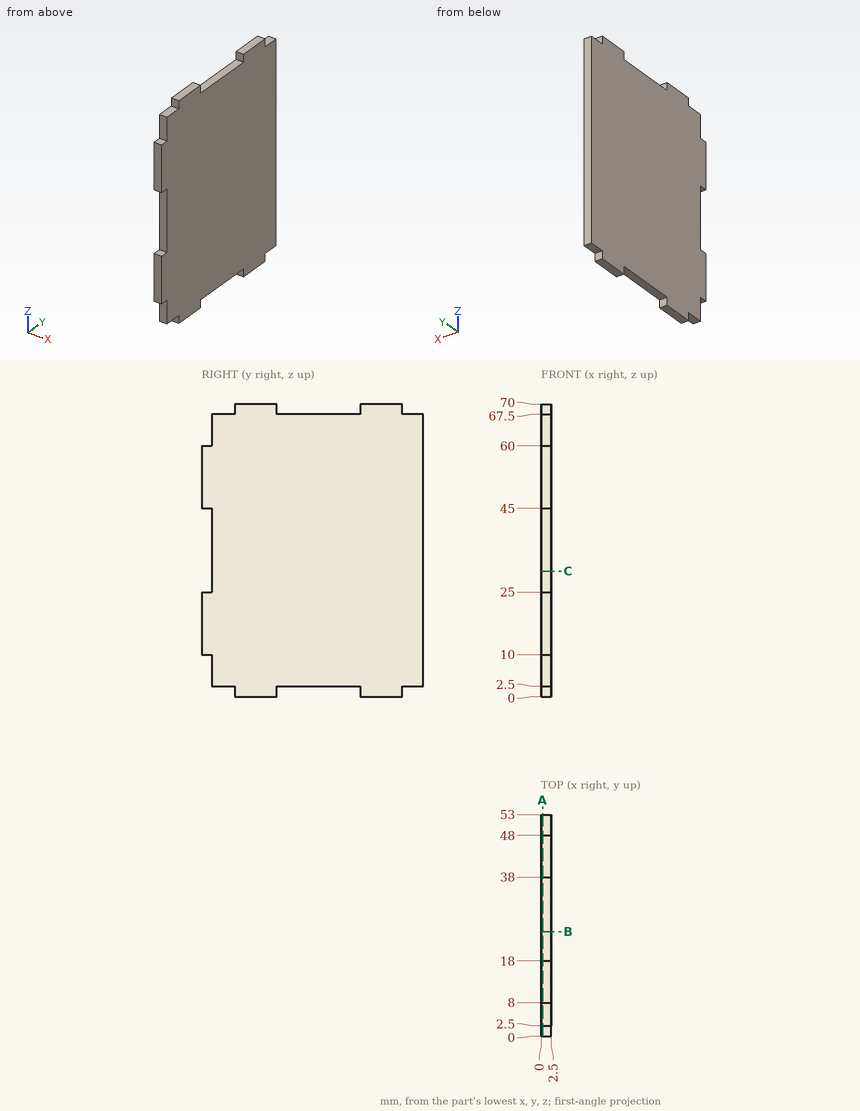
Design review of the part shown in the three views and the two pictorial views. Dimensions are in mm from the part's minimum x, y and z. Give positions to 0.01 mm unless a question says otherwise; leave off trailing zeros. Loops run counter-clockwise (first coordinate to the right, second up) from the corner with the lowest first, then second, coordinate; pieces in that order, holes last. Notation, with made-up numbers: M -15.5,85 L 3.5,85 A15 cw 3.5,99 Z; hole C 54.5,-30.75 d8. An arc over 180 degrees is marked long. Put each result on its own line as item: value. Start each with the question number.
(1) For pin 1 (1.2 mm diameter, centred on x = 1.5, z = 68.5, fed in from -Y); pin 2 (0.8 mm diameter, centred on x = 1.5, z = 0.5, fed in from +Y); pin 3 (1.2 mm diameter, centred on x = 1.5, y = 1, fed in from +Z), all flat-tipped, find the tip position at first contact; note any pin that passes through.
(2) Wall thickness on L1, parallel to Z at x = 1.15, y = 29; L2, parallel to Y at x = 1.55, z = 31: over which ranges is each line inside the solid? List them lowest first.
(3) Add section C-C, the plane z = 30. Write out the cut boundary in (x, y), then the cut area to 3 significant figures.
(4) Add section B-B, the plane y = 25. Write out the cut boundary in (x, z), then the cut area to 4 significant figures.
(5) Add section A-A, the plane x = 0.4. Write out the cut boundary in (y, z).
Result:
1. pin 1: stops at y = 8
1. pin 2: stops at y = 48
1. pin 3: stops at z = 60
2. L1: z = 2.5 to 67.5
2. L2: y = 2.5 to 53
3. outline: M 0,2.5 L 2.5,2.5 L 2.5,53 L 0,53 Z
3. area: 126 mm^2
4. outline: M 0,2.5 L 2.5,2.5 L 2.5,67.5 L 0,67.5 Z
4. area: 162.5 mm^2
5. outline: M 0,10 L 2.5,10 L 2.5,2.5 L 8,2.5 L 8,0 L 18,0 L 18,2.5 L 38,2.5 L 38,0 L 48,0 L 48,2.5 L 53,2.5 L 53,67.5 L 48,67.5 L 48,70 L 38,70 L 38,67.5 L 18,67.5 L 18,70 L 8,70 L 8,67.5 L 2.5,67.5 L 2.5,60 L 0,60 L 0,45 L 2.5,45 L 2.5,25 L 0,25 Z
